The listing builds one solid part. Answer for the finished solid, in the listing's coordinates (mm). Face numbers are marked on the shaded views. A direction names the side the tool comes from. Give positions to 0.01 mm unless a question says otherwise; leave off trailing zeros. Write each loop counter-clockwise with the first axis right and the second up, starting at its lowest first coordinate (ties: lowest second). Pieces come first, ordered by that corner, then holes. Notation, with made-up numbers: (23.25, -13.75) - (82.25, -13.75) arc R26 ccw to (82.25, 19.25) - close; hole circle Ø1 at (24, 47). An arc over 180 degrees is marked (long way). Answer as CSV lines item,"result". Start each with the question number.
(1) For a pull along Y with two mould halves and no side action, classify the marked faces 3, 4 and 5 as pulls with the +Y half, pulls with the -Y half, needs draft (parallel to the pull), parting line crosses it, or undercut.
(2) Find section D-D (x = 78.5). Write down the section's boundary in (y, z), then the cut area to 3 significant figures.
(3) Each of these flat-tipped pins is pushed along its axis until it touches: pin 1 Ø14.5 at (y, z) = (15, -162.5) entering from -X; pin 2 Ø1 at (x, z) = (103, -73) entering from -Y; pin 3 Ø5 at (x, z) = (67.7, -5) entering from +Y; pin 4 Ø3 at (x, z) = (4, -165) entering from +Y. Where does it stop, or does it pass through?
(4) Find section C-C (y = 27). Write down the section's boundary in (x, z).
(5) Straight lines are drawn through the part: probe 1 along Z at (x, y) = (116, 2); probe 2 along X at (y, z) = (2.95, -15); probe 3 along Z at (x, y) = (67, 2). For each, find the intervals that lie inside material, in ascending order.
(6) For the marked faces 1 and 2, determine the directions among +Z, -Z, +X, -X, +Y, -Y from which every point of the face is accessible in a straight line to the end or side of a thin tool.
(7) Find section A-A (z = -5). State how many separate pieces and enclosed holes the cut face has, then the cut area to 3 significant figures.
Autodesk Inventor part; units mm, degrees
ref_plane "YZ Plane" through (0, 0, 0) normal (1, 0, 0) x (0, 1, 0)
ref_plane "XZ Plane" through (0, 0, 0) normal (0, 1, 0) x (-1, 0, 0)
ref_plane "XY Plane" through (0, 0, 0) normal (0, 0, 1) x (1, 0, 0)
sketch "Sketch1" plane through (0, 0, 0) normal (1, 0, 0) x (0, 1, 0)
  line L0 (0, 0) -> (40, 0)
  line L1 (40, 0) -> (40, -180)
  line L2 (40, -180) -> (0, -180)
  line L3 (0, -180) -> (0, 0)
  line L4 (0, 0) -> (4, 0)
  line L5 (4, 0) -> (4, -20)
  line L6 (4, -20) -> (0, -20)
  line L7 (0, -20) -> (0, 0)
  line L8 (0, -180) -> (4, -180)
  line L9 (4, -180) -> (4, -160)
  line L10 (4, -160) -> (0, -160)
  line L11 (0, -160) -> (0, -180)
  line L12 (4, -20) -> (4, -56)
  line L13 (4, -160) -> (4, -124)
  line L14 (4, -56) -> (40, -56)
  line L15 (4, -124) -> (40, -124)
  line L16 (40, -124) -> (4, -160)
  line L17 (4, -20) -> (40, -56)
  line L18 (40, -56) -> (36, -56)
  line L19 (36, -56) -> (36, -124)
  line L20 (36, -124) -> (40, -124)
  line L21 (40, -124) -> (40, -56)
  line L22 (4, -20) -> (1.1716, -22.8284)
  line L23 (1.1716, -22.8284) -> (36, -57.6569)
  line L24 (1.1716, -22.8284) -> (0, -21.6569)
  line L25 (4, -160) -> (1.1716, -157.1716)
  line L26 (1.1716, -157.1716) -> (36, -122.3431)
  line L27 (1.1716, -157.1716) -> (-0.2426, -158.5858)
  line L28 (0, 0) -> (40, 0)
  line L29 (40, 0) -> (40, 4)
  line L30 (40, 4) -> (0, 4)
  line L31 (0, 4) -> (0, 0)
  line L32 (40, 0) -> (36, 0)
  line L33 (36, 0) -> (36, -56)
  line L34 (36, -56) -> (40, -56)
  line L35 (40, -56) -> (40, 0)
  line L36 (40, -180) -> (0, -180)
  line L37 (0, -180) -> (0, -184)
  line L38 (0, -184) -> (40, -184)
  line L39 (40, -184) -> (40, -180)
  line L40 (36, -124) -> (40, -124)
  line L41 (40, -124) -> (40, -180)
  line L42 (40, -180) -> (36, -180)
  line L43 (36, -180) -> (36, -124)
  point P0 (0, -158.3431)
  dimension "d0" = 40
  dimension "d1" = 180
  dimension "d2" = 4
  dimension "d3" = 20
  dimension "d4" = 4
  dimension "d5" = 20
  dimension "d6" = 36
  dimension "d7" = 36
  dimension "d8" = 4
  dimension "d9" = 4
  dimension "d10" = 4
  dimension "d67" = 4
  dimension "d68" = 4
extrude "Extrusion1" add sketch "Sketch1" along normal blind 120 contours L31 L30 L29 L0 | L0 L5 L6 L3 | L0 L1 L17 L33 | L17 L14 L33 | L1 L15 L19 L14 | L10 L9 L2 L3 | L16 L43 L15 | L1 L2 L43 L16 | L2 L39 L38 L37
sketch "Sketch2" plane through (0, 4, 0) normal (0, 1, 0) x (1, 0, 0)
  line L0 (0, 0) -> (120, 0)
  line L1 (0, 0) -> (4, 0)
  line L2 (4, 0) -> (4, 5)
  line L3 (4, 5) -> (0, 5)
  line L4 (0, 5) -> (0, 0)
  line L5 (4, 5) -> (4, 15)
  circle A0 centre (4, 15) radius 2
  circle A1 centre (4, 5) radius 2
  line L6 (120, 0) -> (116, 0)
  line L7 (116, 0) -> (116, 5)
  line L8 (116, 5) -> (120, 5)
  line L9 (120, 5) -> (120, 0)
  line L10 (116, 5) -> (116, 15)
  circle A2 centre (116, 15) radius 2
  circle A3 centre (116, 5) radius 2
  line L11 (0, 20) -> (120, 20)
  line L12 (120, 0) -> (112, 0)
  line L13 (112, 0) -> (112, 20)
  line L14 (112, 20) -> (120, 20)
  line L15 (120, 20) -> (120, 0)
  line L16 (0, 0) -> (8, 0)
  line L17 (8, 0) -> (8, 20)
  line L18 (8, 20) -> (0, 20)
  line L19 (0, 20) -> (0, 0)
  line L20 (112, 20) -> (71.7, 20)
  line L21 (71.7, 20) -> (71.7, 0)
  line L22 (71.7, 0) -> (112, 0)
  line L23 (112, 0) -> (112, 20)
  line L24 (8, 20) -> (48.3, 20)
  line L25 (48.3, 20) -> (48.3, 0)
  line L26 (48.3, 0) -> (8, 0)
  line L27 (8, 0) -> (8, 20)
  line L28 (48.3, 0) -> (52.3, 0)
  line L29 (52.3, 0) -> (52.3, 5)
  line L30 (52.3, 5) -> (48.3, 5)
  line L31 (48.3, 5) -> (48.3, 0)
  line L32 (52.3, 5) -> (52.3, 15)
  circle A4 centre (52.3, 15) radius 2
  circle A5 centre (52.3, 5) radius 2
  line L33 (48.3, 20) -> (48.3, 0)
  line L34 (71.7, 0) -> (67.7, 0)
  line L35 (67.7, 0) -> (67.7, 5)
  line L36 (67.7, 5) -> (71.7, 5)
  line L37 (71.7, 5) -> (71.7, 0)
  line L38 (67.7, 5) -> (67.7, 15)
  circle A6 centre (67.7, 15) radius 2
  circle A7 centre (67.7, 5) radius 2
  line L39 (71.7, 20) -> (71.7, 0)
  line L40 (0, 20) -> (120, 20)
  line L41 (120, 20) -> (120, 0)
  line L42 (120, 0) -> (0, 0)
  line L43 (0, 0) -> (0, 20)
  line L44 (0, 180) -> (0, 160)
  line L45 (0, 180) -> (-1.8149, 180)
  line L46 (0, 160) -> (4, 160)
  line L47 (4, 160) -> (4, 165)
  line L48 (4, 165) -> (0, 165)
  line L49 (0, 165) -> (0, 160)
  line L50 (4, 165) -> (4, 175)
  circle A8 centre (4, 175) radius 2
  circle A9 centre (4, 165) radius 2
  line L51 (120, 160) -> (116, 160)
  line L52 (116, 160) -> (116, 165)
  line L53 (116, 165) -> (120, 165)
  line L54 (120, 165) -> (120, 160)
  line L55 (116, 165) -> (116, 175)
  circle A10 centre (116, 175) radius 2
  circle A11 centre (116, 165) radius 2
  line L56 (120, 160) -> (112, 160)
  line L57 (112, 160) -> (112, 180)
  line L58 (112, 180) -> (120, 180)
  line L59 (120, 180) -> (120, 160)
  line L60 (0, 160) -> (8, 160)
  line L61 (8, 160) -> (8, 180)
  line L62 (8, 180) -> (0, 180)
  line L63 (0, 180) -> (0, 160)
  line L64 (112, 180) -> (71.7, 180)
  line L65 (71.7, 180) -> (71.7, 160)
  line L66 (71.7, 160) -> (112, 160)
  line L67 (112, 160) -> (112, 180)
  line L68 (8, 180) -> (48.3, 180)
  line L69 (48.3, 180) -> (48.3, 160)
  line L70 (48.3, 160) -> (8, 160)
  line L71 (8, 160) -> (8, 180)
  line L72 (52.3, 165) -> (52.3, 175)
  circle A12 centre (52.3, 165) radius 2
  circle A13 centre (52.3, 175) radius 2
  line L73 (48.3, 180) -> (48.3, 160)
  line L74 (52.3, 165) -> (48.3, 165)
  line L75 (48.3, 160) -> (52.3, 160)
  line L76 (48.3, 165) -> (48.3, 160)
  line L77 (52.3, 160) -> (52.3, 165)
  line L78 (67.7, 160) -> (67.7, 165)
  line L79 (67.7, 165) -> (67.7, 175)
  circle A14 centre (67.7, 165) radius 2
  circle A15 centre (67.7, 175) radius 2
  line L80 (71.7, 160) -> (67.7, 160)
  line L81 (71.7, 165) -> (71.7, 160)
  line L82 (67.7, 165) -> (71.7, 165)
  line L83 (71.7, 180) -> (71.7, 160)
  line L84 (0, 180) -> (120, 180)
  line L85 (120, 180) -> (120, 160)
  line L86 (120, 160) -> (0, 160)
  line L87 (0, 160) -> (0, 180)
  point P0 (112, 0)
  dimension "d13" = 4
  dimension "d14" = 5
  dimension "d15" = 10
  dimension "d16" = 4
  dimension "d17" = 4
  dimension "d18" = 4
  dimension "d19" = 5
  dimension "d20" = 10
  dimension "d21" = 4
  dimension "d22" = 4
  dimension "d23" = 8
  dimension "d24" = 8
  dimension "d25" = 40.3
  dimension "d26" = 40.3
  dimension "d27" = 4
  dimension "d28" = 5
  dimension "d29" = 10
  dimension "d30" = 4
  dimension "d31" = 4
  dimension "d32" = 4
  dimension "d33" = 5
  dimension "d34" = 10
  dimension "d35" = 4
  dimension "d36" = 4
  dimension "d37" = 4
  dimension "d38" = 5
  dimension "d39" = 10
  dimension "d40" = 4
  dimension "d41" = 4
  dimension "d42" = 4
  dimension "d43" = 5
  dimension "d44" = 10
  dimension "d45" = 4
  dimension "d46" = 4
  dimension "d47" = 8
  dimension "d48" = 8
  dimension "d49" = 40.3
  dimension "d50" = 40.3
  dimension "d51" = 4
  dimension "d52" = 5
  dimension "d53" = 10
  dimension "d54" = 4
  dimension "d55" = 4
  dimension "d56" = 4
  dimension "d57" = 5
  dimension "d58" = 10
  dimension "d59" = 4
  dimension "d60" = 4
extrude "Extrusion2" cut sketch "Sketch2" against normal blind 120 contours A0 | A1 L3 L2 | L2 L5 A1 | A1 L5 L3 | A6 | A4 | A5 L30 L29 | L29 L32 A5 | A5 L32 L30 | A7 L38 L35 | L35 L36 A7 | A2 | L38 A7 L36 | A3 L10 L7 | L7 L8 A3 | L8 L10 A3 | A8 | L68 L69 L70 L61 | A9 L50 L48 | L48 L47 A9 | A13 | A15 | L50 A9 L47 | L64 L57 L66 L65 | L74 L77 A12 | A12 L72 L74 | A10 | L77 L72 A12 | L82 L79 A14 | A14 L78 L82 | A14 L79 L78 | A11 L55 L52 | L52 L53 A11 | L53 L55 A11
sketch "Sketch4" plane through (0, 4, -180) normal (0, 0, 1) x (1, 0, 0)
  line L0 (8, 0) -> (8, -4)
  line L1 (0, 32) -> (120, 32)
  line L2 (8, 0) -> (53, 0)
  line L3 (53, 0) -> (53, 32)
  line L4 (53, 32) -> (8, 32)
  line L5 (8, 32) -> (8, 0)
  line L6 (112, 0) -> (112, -4)
  line L7 (112, 0) -> (67, 0)
  line L8 (67, 0) -> (67, 32)
  line L9 (67, 32) -> (112, 32)
  line L10 (112, 32) -> (112, 0)
  point P0 (0, -4)
  point P1 (67, 32)
  point P2 (8, 32)
  dimension "d69" = 45
  dimension "d70" = 45
fillet "Fillet1" radius 25 2 edges at (60, 36, -180) (60, 36, 0)
fillet "Fillet2" radius 29 2 edges at (60, 40, -184) (60, 40, 4)
extrude "Extrusion4" cut sketch "Sketch4" along normal mid plane 1000
properties part number "back"
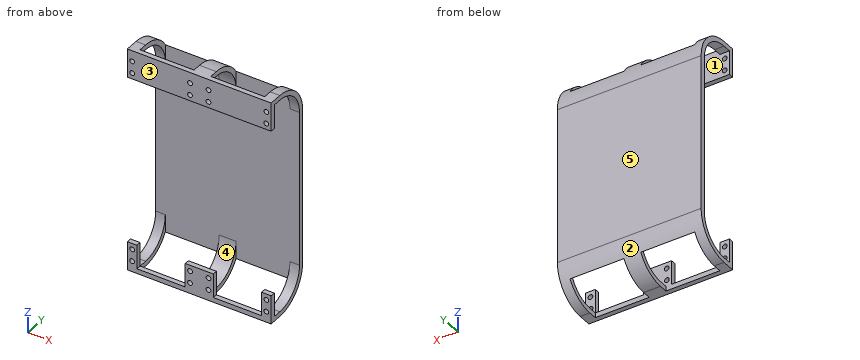
Result set:
1,face 3,"pulls with the -Y half"
1,face 4,"undercut"
1,face 5,"pulls with the +Y half"
2,outline,"(0, -184) - (4, -184) - (4, -180) - (0, -180) - close; (0, -20) - (4, -20) - (4, 4) - (0, 4) - close; (36, -169.7) arc R29 ccw to (40, -155) - (40, -25) arc R29 ccw to (36, -10.3) - close"
2,area,"712 mm^2"
3,pin 1,"through"
3,pin 2,"y = 36"
3,pin 3,"y = 34.05"
3,pin 4,"y = 38.73"
4,outline,"(0, -179.19) - (8, -179.19) - (8, -174.21) - (0, -174.21) - close; (0, -5.79) - (8, -5.79) - (8, -0.81) - (0, -0.81) - close; (53, -179.19) - (67, -179.19) - (67, -174.21) - (53, -174.21) - close; (53, -5.79) - (67, -5.79) - (67, -0.81) - (53, -0.81) - close; (112, -179.19) - (120, -179.19) - (120, -174.21) - (112, -174.21) - close; (112, -5.79) - (120, -5.79) - (120, -0.81) - (112, -0.81) - close"
5,probe 1,"-184 to -177, -173 to -167, -163 to -160, -20 to -17, -13 to -7, -3 to 4"
5,probe 2,"0 to 2, 6 to 50.3, 54.3 to 65.7, 69.7 to 114, 118 to 120"
5,probe 3,"-184 to -176.87, -173.13 to -166.87, -163.13 to -160, -20 to -16.87, -13.13 to -6.87, -3.13 to 4"
6,face 1,"none"
6,face 2,"-Z, +X, -X, +Y"
7,separate pieces,"8"
7,enclosed holes,"0"
7,area,"596 mm^2"
